Check sheet for the modelled part. Datum: model origin and axes. Units: mm. Round coordinates to 2 decimals unless told otherwise and drop trailing zeros. Order: outer loops, then holes, each group sorted by start corner. A loop starts at its lowest first (then second) coordinate and runs counter-clockwise, first axis right, second up.
(1) Sectioned sample at A-A, the plane x = 1206.5. Enter the section's corners in (y, z) (1 decimal).
(2) Depth check by flat-ended pin: pin 1 (8 mm diameter, centred on y = 33.5, z = 38.5, fed in from -X); pin 2 (5.5 mm diameter, centred on x = 1204.5, z = -59, fed in from -Y); pin 3 (0.8 mm diameter, centred on y = 51, z = 53, fed in from -X). Enter the tip coordinate at first touch or a pass-through.
(3) Thickness scan on probe 1 along Y at (x, z) = (1200.5, 213); probe 2 along Y at (x, z) = (1218, 139); probe 3 along Y at (x, z) = (1192.5, 6). Record the ranges inside material, lowest first.
(4) Mould release check, pull along Y, two halves, no side actions. Record for faces 1 (the flat face through (1219.2, 28, 4)), 2 (the flat face through (1209, 49.974, 4)), 3 (the flat face through (1202, 38.1, 4)), 4 (the flat face through (1201, 39.688, 4)): released by +Y, released by -Y, zero draft, split by the parting line, or undercut.
```python
from build123d import *

# Parameters (mm, degrees)
EXTRUDE1_DEPTH = 257.175


with BuildPart() as part:
    # Sketch1 → Extrude1 (new body, symmetric)
    with BuildSketch(Plane.XY):
        with BuildLine():
            Line((1219.2, 19.05), (1219.2, 36.5125))
            ThreePointArc((1219.2, 36.5125), (1218.735032015, 37.635032015), (1217.6125, 38.1))
            Line((1217.6125, 38.1), (1185.2275, 38.1))
            Line((1185.2275, 38.1), (1185.2275, 39.6875))
            Line((1185.2275, 39.6875), (1217.6125, 39.6875))
            ThreePointArc((1217.6125, 39.6875), (1218.735032015, 40.152467985), (1219.2, 41.275))
            Line((1219.2, 41.275), (1219.2, 48.387))
            ThreePointArc((1219.2, 48.387), (1218.735032015, 49.509532015), (1217.6125, 49.9745))
            Line((1217.6125, 49.9745), (1199.5785, 49.9745))
            Line((1199.5785, 49.9745), (1199.5785, 51.562))
            Line((1199.5785, 51.562), (1217.6125, 51.562))
            ThreePointArc((1217.6125, 51.562), (1219.85756403, 50.63206403), (1220.7875, 48.387))
            Line((1220.7875, 48.387), (1220.7875, 19.05))
            Line((1220.7875, 19.05), (1219.2, 19.05))
        make_face()
    extrude(amount=EXTRUDE1_DEPTH, both=True)


solid = part.part
```
Derived:
1. outline: (38.1, -257.2) - (39.7, -257.2) - (39.7, 257.2) - (38.1, 257.2) - close; (50, -257.2) - (51.6, -257.2) - (51.6, 257.2) - (50, 257.2) - close
2. pin 1: stops at x = 1218.86
2. pin 2: stops at y = 38.1
2. pin 3: stops at x = 1199.58
3. probe 1: y = 38.1 to 39.69, 49.97 to 51.56
3. probe 2: y = 38.05 to 39.74, 49.93 to 51.54
3. probe 3: y = 38.1 to 39.69
4. face 1: zero draft
4. face 2: undercut
4. face 3: released by -Y
4. face 4: undercut
